from build123d import *

# Parameters (mm, degrees)
SKETCH2_W           = 140
SKETCH2_H           = 60
BOSS_EXTRUDE2_DEPTH = 5
SKETCH3_W           = 140
SKETCH3_H           = 5
BOSS_EXTRUDE3_DEPTH = 50
SKETCH4_R           = 7
CUT_EXTRUDE1_DEPTH  = 108.354552768
SKETCH6_W           = 50
SKETCH6_H           = 50
SKETCH6_W_2         = 40
SKETCH6_H_2         = 40
SKETCH7_R           = 7
BOSS_EXTRUDE4_DEPTH = 5
SKETCH8_W           = 140
SKETCH8_H           = 50
CUT_EXTRUDE2_DEPTH  = 5


with BuildPart() as part:
    # Sketch2 → Boss-Extrude2 (new body)
    with BuildSketch(Plane(origin=(0, 0, 0), x_dir=(1, 0, 0), z_dir=(0, 1, 0))):
        Rectangle(SKETCH2_W, SKETCH2_H)
    extrude(amount=-BOSS_EXTRUDE2_DEPTH)

    # Sketch3 → Boss-Extrude3 (add)
    with BuildSketch(Plane.XZ.offset(5)):
        with Locations((0, -27.5)):
            Rectangle(SKETCH3_W, SKETCH3_H)
        with Locations((0, 27.5)):
            Rectangle(SKETCH3_W, SKETCH3_H)
    extrude(amount=BOSS_EXTRUDE3_DEPTH)

    # Sketch4 → Cut-Extrude1 (cut, through all)
    with BuildSketch(Plane(origin=(0, 0, -30), x_dir=(-1, 0, 0), z_dir=(0, 0, -1))):
        with Locations((-52.5, -27.5)):
            Circle(SKETCH4_R)
        with Locations((52.5, -27.5)):
            Circle(SKETCH4_R)
    extrude(amount=-CUT_EXTRUDE1_DEPTH, mode=Mode.SUBTRACT)

    # Sweep1: sweep along a path in Sketch5
    with BuildLine(Plane.XY) as sweep1_path:
        Line((0, 0), (0, 460))
        ThreePointArc((0, 460), (41.005050634, 558.994949366), (140, 600))
        Line((140, 600), (350, 600))
    # Sketch6 → Sweep1 (sweep)
    with BuildSketch(Plane(origin=(0, 0, 0), x_dir=(1, 0, 0), z_dir=(0, 1, 0))):
        Rectangle(SKETCH6_W, SKETCH6_H)
        Rectangle(SKETCH6_W_2, SKETCH6_H_2, mode=Mode.SUBTRACT)
    sweep(path=sweep1_path.line)

    # Sketch7 → Boss-Extrude4 (add)
    with BuildSketch(Plane(origin=(350, 0, 0), x_dir=(0, 0, -1), z_dir=(1, 0, 0))):
        with BuildLine():
            Line((-25, 550), (-25, 650))
            ThreePointArc((-25, 650), (0, 675), (25, 650))
            Line((25, 650), (25, 550))
            ThreePointArc((25, 550), (0, 525), (-25, 550))
        make_face()
        with Locations(Location((0, 650, 0), (0, 0, 90))):
            Circle(SKETCH7_R, mode=Mode.SUBTRACT)
        with Locations(Location((0, 550, 0), (0, 0, 270))):
            Circle(SKETCH7_R, mode=Mode.SUBTRACT)
    extrude(amount=BOSS_EXTRUDE4_DEPTH)

    # Sketch8 → Cut-Extrude2 (cut)
    with BuildSketch(Plane(origin=(0, 0, -30), x_dir=(-1, 0, 0), z_dir=(0, 0, -1))):
        with Locations((0, -30)):
            Rectangle(SKETCH8_W, SKETCH8_H)
    extrude(amount=-CUT_EXTRUDE2_DEPTH, mode=Mode.SUBTRACT)


solid = part.part
The listing builds one solid part. Answer for the finished solid, in the listing's coordinates (mm). A direction names the side the tool comes from. Give positions to 0.01 mm unless a question says otherwise; leave off trailing zeros. Order: outer loops, then holes, each group sorted by start corner. A loop starts at its lowest first (then second) coordinate and runs counter-clockwise, first axis right, second up. Notation, with made-up numbers: (45, 18) -> (98, 18) arc R26 ccw to (98, 42) -> close; hole circle Ø4 at (44, 82). An arc over 180 degrees is marked (long way). Put each result on its own line as item: value.
Item 1: For faces 1 (the face through (350, 556, 5)), 2 (the face through (54.219, 543.915, 0.28)), 3 (the face through (350, 644.8, 5.2)), 4 (the face through (70, -3, 13)), determine the directions among +Z, -Z, +X, -X, +Y, -Y from which every point of the face is accessible in a straight line to the end or side of a thin tool.
Established:
face 1: +Z, -Z, -Y
face 2: none
face 3: +Z, -Z, -X, +Y
face 4: +Z, -Z, +X, -Y
Item 2: A cutting plane is placed at C-C on x = -52.5. Give the vertices of the cut face in (y, z), plus the area to 3 significant figures.
Established:
outline: (-55, 25) -> (-34.5, 25) -> (-34.5, 30) -> (-55, 30) -> close; (-20.5, 25) -> (-5, 25) -> (-5, -30) -> (0, -30) -> (0, 30) -> (-20.5, 30) -> close
area: 480 mm^2
Item 3: For a pull along Y with two mould halves and no side action, classify faces 5 (the face through (355, 601, 0)), 6 (the face through (-55.73, -33.71, 27.47)), 7 (the face through (246, 575, 0)) as released by +Y, released by -Y, zero draft, split by the parting line, or undercut.
Established:
face 5: zero draft
face 6: undercut
face 7: released by -Y
Item 4: A cutting plane is placed at A-A on z = 0. Count the separate pieces of the cut face and the enclosed holes in it, plus the area to 3 significant figures.
Established:
separate pieces: 3
enclosed holes: 1
area: 10,200 mm^2
Item 5: Given P1, Ø3, axis at x = 134, z = -10, coming from the +Y side; P2, Ø12, axis at y = 302.5, z = -14.5, coming from the +X side; P3, Ø22.5, axis at x = -52.5, y = -27.5, coming from the -Z side; P4, Ø22.5, axis at x = 52.5, y = -27.5, coming from the +Z side, each flat-ended and moving along its own axis, determine where each tip first touches the part or whether it passes through.
Established:
P1: stops at y = 624.94
P2: stops at x = 25
P3: stops at z = 25
P4: stops at z = 30
Item 6: Straight lines are drawn through the part: line 1 (X direction, y = -27, z = 27); line 2 (X direction, y = 319.5, z = 13.5); line 3 (Y direction, x = -52, z = 26). For each, find the intervals that lie inside material, in ascending order.
Established:
line 1: x = -70 to -59.48, -45.52 to 45.52, 59.48 to 70
line 2: x = -25 to -20, 20 to 25
line 3: y = -55 to -34.48, -20.52 to 0
Item 7: A cutting plane is placed at D-D on x = 52.5. Give the vertices of the cut face in (y, z), plus the area to 3 significant figures.
Established:
outline: (-55, 25) -> (-34.5, 25) -> (-34.5, 30) -> (-55, 30) -> close; (-20.5, 25) -> (-5, 25) -> (-5, -30) -> (0, -30) -> (0, 30) -> (-20.5, 30) -> close; (534.62, -25) -> (599.89, -25) -> (599.89, 25) -> (534.62, 25) -> close; hole (542.12, -20) -> (593.95, -20) -> (593.95, 20) -> (542.12, 20) -> close
area: 1,670 mm^2
Item 8: A cutting plane is placed at B-B on y = -27.5. Give the vertices of the cut face in (x, z).
Established:
outline: (-70, 25) -> (-59.5, 25) -> (-59.5, 30) -> (-70, 30) -> close; (-45.5, 25) -> (45.5, 25) -> (45.5, 30) -> (-45.5, 30) -> close; (59.5, 25) -> (70, 25) -> (70, 30) -> (59.5, 30) -> close
